Check sheet for the drawn part. Datum: minimum x, y, z corner. Units: mm. A direction names the side the tool comes from. Coordinates: 2 decimals unless noted, no trailing zeros. Write each loop counter-clockwise with the first axis right and the second up, starting at its lowest first coordinate (ties: lowest second). Pieces come first, ordered by that corner, then holes. Notation, with made-up numbers: (45, -29.75) -> (94, -29.75) arc R13 cw to (94, -6.75) -> close; hole circle Ø11 at (-33, -4.5). An arc over 180 degrees is marked (long way). One line per question, with ' | ' between items.
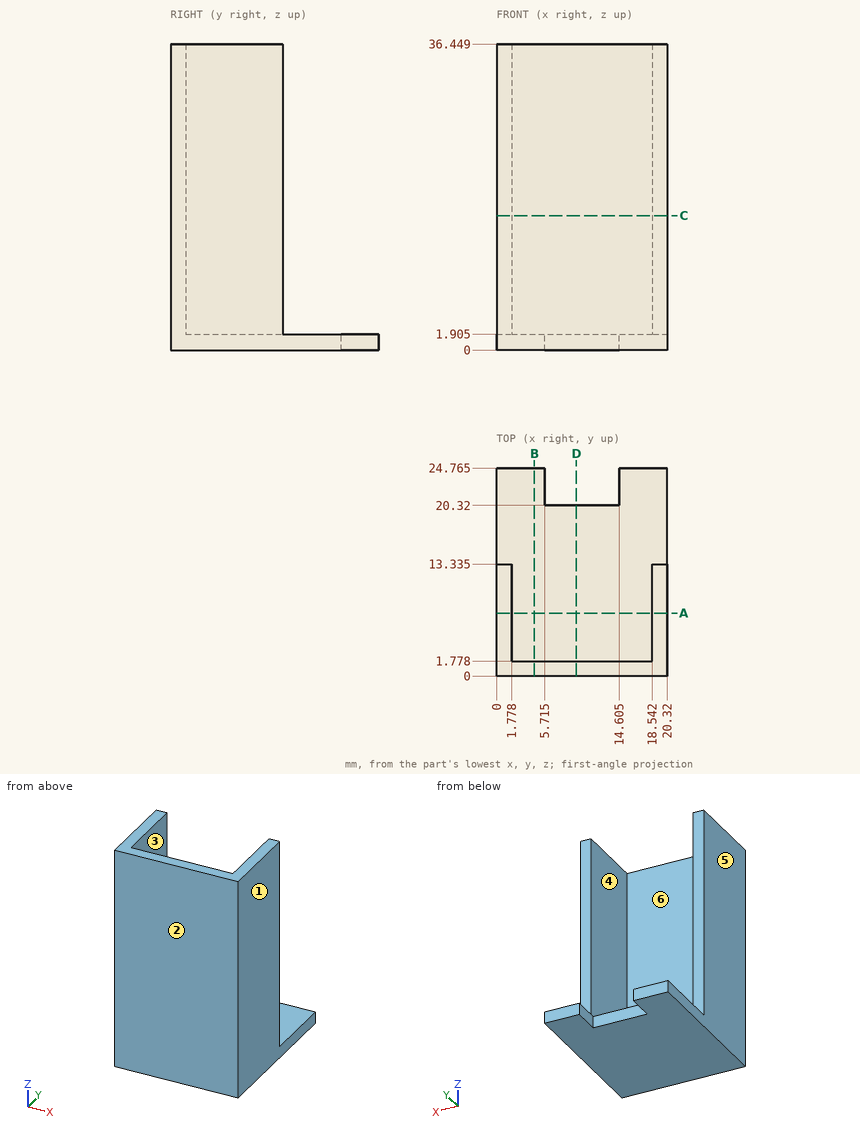
1. Cross-section at D-D on x = 9.5. Record the boundary of the cut face in (y, z) (3 decimals).
Worked answers:
outline: (0, 0) -> (20.32, 0) -> (20.32, 1.905) -> (1.778, 1.905) -> (1.778, 36.449) -> (0, 36.449) -> close
2. Material ranges on line 1 (X direction, y = 7, z = 20.5); line 2 (Y direction, x = 10.5, z = 5.5); line 3 (Z direction, x = 5.5, y = 21.25) (3 decimals), recorded low to high. Write a range as from..to.
Worked answers:
line 1: 0..1.78, 18.54..20.32 | line 2: 0..1.78 | line 3: 0..1.905
3. Cross-section at C-C on z = 16. Record the boundary of the cut face in (x, y) (3 decimals).
Worked answers:
outline: (0, 0) -> (20.32, 0) -> (20.32, 13.335) -> (18.542, 13.335) -> (18.542, 1.778) -> (1.778, 1.778) -> (1.778, 13.335) -> (0, 13.335) -> close
4. Go/stop test with flat-tipped pins: P1, Ø1, axis at x = 17, y = 19, coming from the +Z side (3 decimals); P2, Ø1.5, axis at x = 17.5, z = 23.5, coming from the +Y side; P3, Ø2, axis at x = 10, z = 1, coming from the +Y side. Record where each tip stops, or that it passes through.
Worked answers:
P1: z = 1.905 | P2: y = 1.78 | P3: y = 20.32
5. Tool access check on the marked faces 5 and 6. Record the directions out of +Z, -Z, +X, -X, +Y, -Y that give a thin tool (end or side, any length) a straight path to the whole face; none if there is none.
Worked answers:
face 5: +Z, -Z, -X, +Y, -Y | face 6: +Z, +Y
6. Cross-section at B-B on x = 4.5. Record the boundary of the cut face in (y, z) (3 decimals).
Worked answers:
outline: (0, 0) -> (24.765, 0) -> (24.765, 1.905) -> (1.778, 1.905) -> (1.778, 36.449) -> (0, 36.449) -> close
7. Mould release check, pull along X, two halves, no side actions. Record for the marked faces 1, 2, 3 and 4: released by +X, released by -X, zero draft, split by the parting line, or undercut.
Worked answers:
face 1: released by +X | face 2: zero draft | face 3: undercut | face 4: undercut
8. Cross-section at A-A on y = 7.5. Record the boundary of the cut face in (x, z) (3 decimals), and give its area (3 significant figures).
Worked answers:
outline: (0, 0) -> (20.32, 0) -> (20.32, 36.449) -> (18.542, 36.449) -> (18.542, 1.905) -> (1.778, 1.905) -> (1.778, 36.449) -> (0, 36.449) -> close | area: 162 mm²
